Model file for the job. Use its own axes, mm. Round coordinates to 2 decimals unless told otherwise and drop trailing zeros. Loops run counter-clockwise (first coordinate to the right, second up) from the corner with the lowest first, then second, coordinate; pieces in that order, holes last.
from build123d import *

# Parameters (mm, degrees)
F1_DEPTH = 18


with BuildPart() as f1:
    # F0 (on Front) → F1 (new body)
    with BuildSketch(Plane.XZ):
        Polygon((100, -100), (310, -100), (100, 200), align=None)
        Polygon((-310, -200), (-100, -200), (100, -200), (310, -200), (310, -100), (100, -100), (100, 200), (-100, 200), (-100, -100), (-310, -100), align=None)
        Polygon((-100, 200), (-310, -100), (-100, -100), align=None)
    extrude(amount=F1_DEPTH)


solid = f1.part
Q1. Slice it at C-C on x = 208.5. Give the cut face in (y, z), plus the area to 3 significant figures.
Q2. Flat gauge pins, fed straight in: P1, Ø10, axis at y = -7, z = 136.5, coming from the +X side; P2, Ø10, axis at y = -10.5, z = 71.5, coming from the -X side; P3, Ø4, axis at x = -126, y = -13.5, coming from the +Z side. Where does each tip first touch, or does it go through?
Q3. Slice it at A-A on y = -9.75. Give the cut face in (x, z).
Q4. Probe line 1 (X direction, y = -14, z = -6.5); line 2 (X direction, y = -16.25, z = 18); line 3 (Z direction, x = -257, y = -7). List the from-to ranges inside material, lowest first.
Q5. Slice it at B-B on z = 20.5. Give the cut face in (x, y), plus the area to 3 significant figures.
Reply:
1. outline: (-18, -200) - (0, -200) - (0, 45) - (-18, 45) - close
1. area: 4,410 mm2
2. P1: stops at x = 147.95
2. P2: stops at x = -193.45
2. P3: stops at z = 165.71
3. outline: (-310, -200) - (310, -200) - (310, -100) - (100, 200) - (-100, 200) - (-310, -100) - close
4. line 1: x = -244.55 to 244.55
4. line 2: x = -227.4 to 227.4
4. line 3: z = -200 to -24.29
5. outline: (-225.65, -18) - (225.65, -18) - (225.65, 0) - (-225.65, 0) - close
5. area: 8,120 mm2
